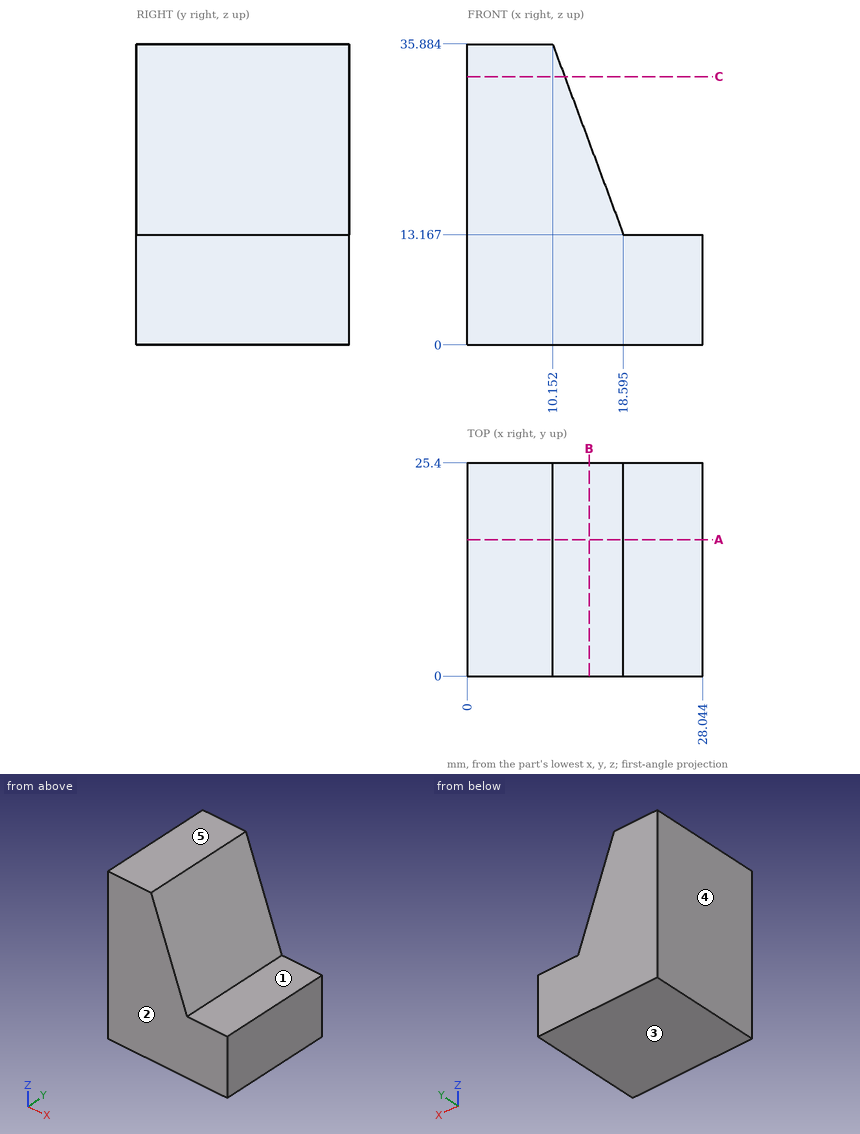
Source: three-view drawing plus pictorial views. Frame: mm from the lowest corner of the part. A direction names the side the tool comes from. Coordinates: 2 decimals unless noted, no trailing zeros. Loops run counter-clockwise (first coordinate to the right, second up) from the corner with the lowest first, then second, coordinate; pieces in that order, holes last. Notation, with made-up numbers: (75.25, 11.5) -> (99.25, 11.5) arc R20 ccw to (99.25, 29.5) -> close; hole circle Ø2 at (14, -24). An arc over 180 degrees is marked (long way). Answer in a Markdown table with one row per item. Add a question column.
Q1. Section C-C on z = 32. Return the cut outline in (x, y) (1 decimal).
Q2. Section A-A on y = 16.25. Return the cut outline in (x, z) (1 decimal).
Q3. Contact query for flat-ended pins moving along their axis: pin 1 Ø10 at (y, z) = (17.5, 22.5) entering from +X (1 decimal); pin 2 Ø3 at (y, z) = (7, 15) entering from +X. Output: stop coordinate, or through.
Q4. Pull-direction query (Z, two-part tool) for the marked faces 3, 4 and 5; classes: pulls with the +Z half, pulls with the -Z half, needs draft (parallel to the pull), parting line crosses it, or undercut.
Q5. Reachability of the marked faces 1 and 2 from +Z, -Z, +X, -X, +Y, -Y: full face, straight path, thin tool, end or side. Return the list, or none.
Q6. Section B-B on x = 14.5. Return the cut outline in (y, z) (1 decimal), and give its area (3 significant figures).
Q7. Ray query, line 1 along Z through (x, y) = (21.25, 10.75); line 2 along X through (y, z) = (4.75, 25); line 3 along X through (y, z) = (18, 31.5). Return the intervals inside material, ascending.
Computed values:
| question | item | result |
|---|---|---|
| 1 | outline | (0, 0) -> (11.6, 0) -> (11.6, 25.4) -> (0, 25.4) -> close |
| 2 | outline | (0, 0) -> (28, 0) -> (28, 13.2) -> (18.6, 13.2) -> (10.2, 35.9) -> (0, 35.9) -> close |
| 3 | pin 1 | stops at x = 17 |
| 3 | pin 2 | stops at x = 18.47 |
| 4 | face 3 | pulls with the -Z half |
| 4 | face 4 | needs draft |
| 4 | face 5 | pulls with the +Z half |
| 5 | face 1 | +Z, +X, +Y, -Y |
| 5 | face 2 | +Z, -Z, +X, -X, -Y |
| 6 | outline | (0, 0) -> (25.4, 0) -> (25.4, 24.2) -> (0, 24.2) -> close |
| 6 | area | 614 mm^2 |
| 7 | line 1 | z = 0 to 13.17 |
| 7 | line 2 | x = 0 to 14.2 |
| 7 | line 3 | x = 0 to 11.78 |
